Model file for the job. Use its own axes, mm. A direction names the side the tool comes from. Give positions to 0.01 mm unless a question says otherwise; leave off trailing zeros. Write each loop counter-clockwise with the first axis right and the second up, starting at its lowest first coordinate (ties: lowest second). Pieces come first, ordered by that corner, then holes.
```python
from build123d import *

# Parameters (mm, degrees)
SKETCH1_W           = 114.3
SKETCH1_H           = 152.4
BOSS_EXTRUDE1_DEPTH = 25.4
CUT_EXTRUDE1_DEPTH  = 99.578509321


with BuildPart() as part:
    # Sketch1 → Boss-Extrude1 (new body)
    with BuildSketch(Plane.XY):
        Rectangle(SKETCH1_W, SKETCH1_H)
    extrude(amount=BOSS_EXTRUDE1_DEPTH)

    # Sketch2 → Cut-Extrude1 (cut, through all)
    with BuildSketch(Plane.XY.offset(25.4)):
        with BuildLine():
            Line((57.15, 71.12), (43.18, 71.12))
            Line((43.18, 71.12), (22.86, 71.12))
            ThreePointArc((22.86, 71.12), (21.063948776, 70.376051224), (20.32, 68.58))
            Line((20.32, 68.58), (20.32, -30.226))
            ThreePointArc((20.32, -30.226), (19.576051224, -32.022051224), (17.78, -32.766))
            Line((17.78, -32.766), (-57.15, -32.766))
            Line((-57.15, -32.766), (-57.15, -76.2))
            Line((-57.15, -76.2), (57.15, -76.2))
            Line((57.15, -76.2), (57.15, 71.12))
        make_face()
        with BuildLine():
            ThreePointArc((15.24, 73.66), (15.983948776, 75.456051224), (17.78, 76.2))
            Line((17.78, 76.2), (-57.15, 76.2))
            Line((-57.15, 76.2), (-57.15, -27.6098))
            Line((-57.15, -27.6098), (12.7, -27.6098))
            ThreePointArc((12.7, -27.6098), (14.496051224, -26.865851224), (15.24, -25.0698))
            Line((15.24, -25.0698), (15.24, 73.66))
        make_face()
    extrude(amount=-CUT_EXTRUDE1_DEPTH, mode=Mode.SUBTRACT)


solid = part.part
```
1. Which spindle directions (+Z, -Z, +X, -X, +Y, -Y) get a long thin tool onto all of the face, cutting with end or side? Do faces 1 (the flat face through (17, 14, 0)), 2 (the flat face through (15.24, 24, 13)), 3 (the flat face through (40, 71.12, 13)). Say none if no direction does.
Calculated:
face 1: -Z, +X, -X, +Y, -Y
face 2: +Z, -Z, -X, +Y
face 3: +Z, -Z, +X, -Y
2. Pin check, flat tips, straight feed: P1, Ø2, axis at x = -27, z = 13, coming from the +Y side; P2, Ø8, axis at x = 19.5, y = 1.5, coming from the -Z side; P3, Ø1.5, axis at y = 32, z = 8.5, coming from the -X side. Stop position of each tip, or through.
Calculated:
P1: stops at y = -27.61
P2: stops at z = 0
P3: stops at x = 15.24
3. Slice it at B-B, the plane y = -2. Write the cut outline in (x, z), and give its area (3 significant figures).
Calculated:
outline: (15.24, 0) - (20.32, 0) - (20.32, 25.4) - (15.24, 25.4) - close
area: 129 mm2
4. Slice it at A-A, the plane z = 12.25. Write the cut outline in (x, y), and give its area (3 significant figures).
Calculated:
outline: (-57.15, -32.77) - (17.78, -32.77) arc R2.54 ccw to (20.32, -30.23) - (20.32, 68.58) arc R2.54 cw to (22.86, 71.12) - (57.15, 71.12) - (57.15, 76.2) - (17.78, 76.2) arc R2.54 ccw to (15.24, 73.66) - (15.24, -25.07) arc R2.54 cw to (12.7, -27.61) - (-57.15, -27.61) - close
area: 1,110 mm2
5. Probe probe 1 along X at (y, z) = (18, 16.5); probe 2 along Y at (x, z) = (-38, 8.5); probe 3 along Y at (x, z) = (49.5, 1.75). List the from-to ranges inside material, lowest first.
Calculated:
probe 1: x = 15.24 to 20.32
probe 2: y = -32.77 to -27.61
probe 3: y = 71.12 to 76.2
6. Slice it at C-C, the plane x = -35. Write the cut outline in (y, z), and give its area (3 significant figures).
Calculated:
outline: (-32.77, 0) - (-27.61, 0) - (-27.61, 25.4) - (-32.77, 25.4) - close
area: 131 mm2
